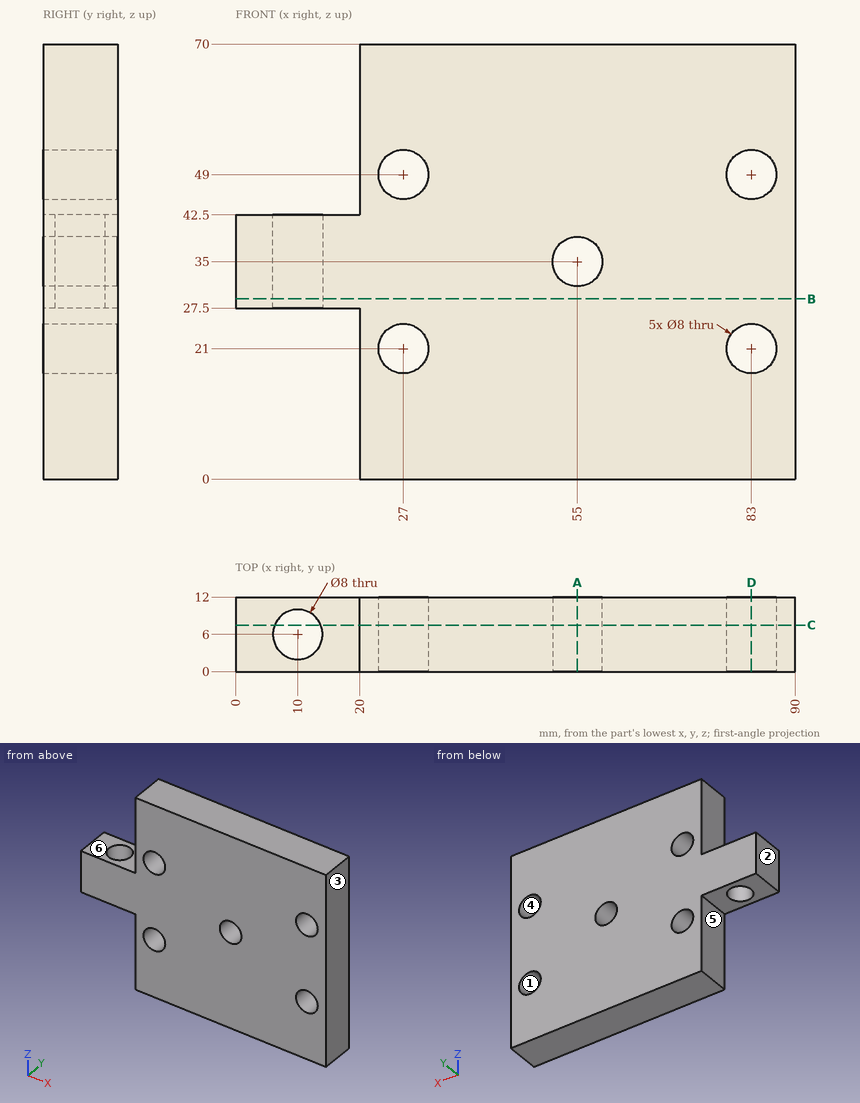
Source: three-view drawing plus pictorial views. Frame: mm from the lowest corner of the part. A direction names the side the tool comes from. Give positions to 0.01 mm unless a question says otherwise; leave off trailing zeros. Order: outer loops, then holes, each group sorted by start corner. A loop starts at its lowest first (then second) coordinate and runs counter-clockwise, first axis right, second up. Notation, with made-up numbers: (76, -34.75) - (80, -34.75) arc R15 ccw to (80, -8.75) - close; hole circle Ø11 at (-15.5, -31). An arc over 180 degrees is marked (long way). Put each result on its own line as item: value.
Item 1: Section query A-A, the plane x = 55. Return loops of the section in (y, z).
Found:
outline: (0, 0) - (12, 0) - (12, 31) - (0, 31) - close; (0, 39) - (12, 39) - (12, 70) - (0, 70) - close
Item 2: Draft query along X for the marked faces 1, 2 and 3. Return one class per face: +X half, -X half, draft (parallel to the pull), parting line (faces both ways), or undercut.
Found:
face 1: undercut
face 2: -X half
face 3: +X half
Item 3: Section query D-D, the plane x = 83. Return loops of the section in (y, z), then the cut area to 3 significant figures.
Found:
outline: (0, 0) - (12, 0) - (12, 17) - (0, 17) - close; (0, 25) - (12, 25) - (12, 45) - (0, 45) - close; (0, 53) - (12, 53) - (12, 70) - (0, 70) - close
area: 648 mm^2
Item 4: Section query B-B, the plane z = 29. Return loops of the section in (x, y).
Found:
outline: (0, 0) - (90, 0) - (90, 12) - (0, 12) - close; hole circle Ø8 at (10, 6)
Item 5: Ray query, L1, parallel to Z at x = 27, y = 4.25; L2, parallel to X at y = 6.75, z = 21; L3, parallel to X at y = 4.5, z = 35. Return the intervals inside material, ascending. Write a range as from..to.
Found:
L1: z = 0..17, 25..45, 53..70
L2: x = 20..23, 31..79, 87..90
L3: x = 0..6.29, 13.71..51, 59..90
Item 6: Section query C-C, the plane y = 7.5. Return loops of the section in (x, z).
Found:
outline: (0, 27.5) - (6.29, 27.5) - (6.29, 42.5) - (0, 42.5) - close; (13.71, 27.5) - (20, 27.5) - (20, 0) - (90, 0) - (90, 70) - (20, 70) - (20, 42.5) - (13.71, 42.5) - close; hole circle Ø8 at (27, 21); hole circle Ø8 at (27, 49); hole circle Ø8 at (55, 35); hole circle Ø8 at (83, 21); hole circle Ø8 at (83, 49)
Item 7: Contact query for flat-ended pins moving along their axis: pin 1 (3.5 mm diameter, centred on y = 3.5, z = 9, fed in from -X); pin 2 (3.5 mm diameter, centred on x = 6.5, y = 8.5, fed in from +Z). Output: stop coordinate, or through.
Found:
pin 1: stops at x = 20
pin 2: stops at z = 42.5
Item 8: Access query for the marked faces 4, 5 and 6. Directions: +Z, -Z, +X, -X, +Y, -Y. A direction counts if a zero-diameter tool reaches every point of the face in a straight line with its end or side. Return the directions, or none.
Found:
face 4: +Y, -Y
face 5: -Z, -X, +Y, -Y
face 6: +Z, -X, +Y, -Y
